Build history of the part. All positions in model axes, mm. A direction names the side the tool comes from. Give positions to 0.01 mm unless a question says otherwise; leave off trailing zeros. Write each loop counter-clockwise with the first axis right and the second up, starting at its lowest first coordinate (ties: lowest second). Pieces come first, ordered by that corner, then holes.
Autodesk Inventor part; units mm, degrees
ref_plane "YZ Plane" through (0, 0, 0) normal (1, 0, 0) x (0, 1, 0)
ref_plane "XZ Plane" through (0, 0, 0) normal (0, 1, 0) x (-1, 0, 0)
ref_plane "XY Plane" through (0, 0, 0) normal (0, 0, 1) x (1, 0, 0)
sketch "Sketch1" plane through (0, 0, 0) normal (0, 1, 0) x (-1, 0, 0)
  line L0 (-4, 0) -> (-157, 0)
  line L1 (-161, -4) -> (-161, -55)
  line L2 (-157, -59) -> (-4, -59)
  line L3 (0, -55) -> (0, -4)
  line L4 (-17, -3.5) -> (-62.5, -3.5)
  line L5 (-62.5, -3.5) -> (-62.5, -9.5)
  line L6 (-62.5, -9.5) -> (-17, -9.5)
  line L7 (-17, -9.5) -> (-17, -3.5)
  line L8 (-38, -15) -> (-64, -15)
  line L9 (-64, -15) -> (-64, -30)
  line L10 (-64, -30) -> (-38, -30)
  line L11 (-38, -30) -> (-38, -15)
  arc A0 (0, -4) -> (-4, 0) centre (-4, -4) ccw
  arc A1 (-157, 0) -> (-161, -4) centre (-157, -4) ccw
  arc A2 (-161, -55) -> (-157, -59) centre (-157, -55) ccw
  arc A3 (-4, -59) -> (0, -55) centre (-4, -55) ccw
  point P0 (0, 0)
  point P1 (-161, 0)
  point P2 (0, -59)
  dimension "d0" = 161
  dimension "d1" = 59
  dimension "d2" = 6
  dimension "d3" = 45.5
  dimension "d4" = 26
  dimension "d5" = 15
  dimension "d6" = 3.5
  dimension "d7" = 15
  dimension "d8" = 17
  dimension "d9" = 38
  dimension "d10" = 4
  dimension "d20" = 51
  dimension "d21" = 153
extrude "Extrusion1" add sketch "Sketch1" along normal blind 4.5
sketch "Sketch2" plane through (0, 4.5, 0) normal (0, 1, 0) x (1, 0, 0)
  line L0 (38, 15) -> (38, 30) construction
  line L1 (38, 30) -> (64, 30) construction
  line L2 (64, 30) -> (64, 15) construction
  line L3 (64, 15) -> (38, 15) construction
  line L4 (17, 3.5) -> (17, 9.5) construction
  line L5 (17, 9.5) -> (62.5, 9.5) construction
  line L6 (62.5, 9.5) -> (62.5, 3.5) construction
  line L7 (62.5, 3.5) -> (17, 3.5) construction
  line L8 (4, 0) -> (157, 0) construction
  arc A0 (157, 0) -> (161, 4) centre (157, 4) ccw construction
  line L9 (161, 4) -> (161, 55) construction
  arc A1 (161, 55) -> (157, 59) centre (157, 55) ccw construction
  line L10 (157, 59) -> (4, 59) construction
  arc A2 (4, 59) -> (0, 55) centre (4, 55) ccw construction
  line L11 (0, 55) -> (0, 4) construction
  arc A3 (0, 4) -> (4, 0) centre (4, 4) ccw construction
  point P0 (0, 0)
hole "Hole1" at (4, 4.5, -55) at (4, 4.5, -4) at (157, 4.5, -4) at (157, 4.5, -55) direction (0, -1, 0) diameter 3.5 end through all
properties part number "A8-0005"
(1) 3-axis set-ups, long thin cutter, end or side, ignore diameter. For faces 5 (the face through (82, 0, -29)), 6 (the face through (40, 2, -9.5)): which of +Z, -Z, +X, -X, +Y, -Y reach the whole face in a straight line?
(2) Saw through at C-C, the plane y = 1.2. List the corners of the cut face in (x, z), plus the area to 3 significant figures.
(3) Saw through at D-D, the plane x = 30.5. List the corners of the cut face in (y, z), plus the area to 4 significant figures.
(4) Mould opens along Z. For faces 1 (the face through (156.474, 2.218, -53.331)), 2 (the face through (39, 2, -3.5)), 3 (the face through (0, 2, -30)), 4 (the face through (159.797, 2.218, -57.859)) say: +Z half, -Z half, draft (parallel to the pull), parting line (faces both ways), or undercut.
(5) Probe line 1 (X direction, y = 2.6, z = -55); line 2 (Z direction, x = 4, y = 2.9); line 3 (X direction, y = 1.75, z = -4). List the from-to ranges inside material, lowest first.
(6) Saw through at B-B, the plane z = -24. List the corners of the cut face in (x, y), plus the area to 4 significant figures.
(7) Saw through at A-A, the plane x = 60. List the corners of the cut face in (y, z), plus the area to 3 significant figures.
(8) Drop a flat-ended pin along its axis: pin 1 (3 mm diameter, centred on x = 157, z = -55, fed in from -Y). Give the stop position or say it passes through.
Computed values:
1. face 5: +Z, -Z, +X, -X, -Y
1. face 6: +Y, -Y
2. outline: (0, -55) arc R4 ccw to (4, -59) - (157, -59) arc R4 ccw to (161, -55) - (161, -4) arc R4 ccw to (157, 0) - (4, 0) arc R4 ccw to (0, -4) - close; hole circle Ø3.5 at (4, -55); hole circle Ø3.5 at (4, -4); hole (17, -9.5) - (62.5, -9.5) - (62.5, -3.5) - (17, -3.5) - close; hole (38, -30) - (64, -30) - (64, -15) - (38, -15) - close; hole circle Ø3.5 at (157, -55); hole circle Ø3.5 at (157, -4)
2. area: 8,780 mm2
3. outline: (0, -59) - (4.5, -59) - (4.5, -9.5) - (0, -9.5) - close; (0, -3.5) - (4.5, -3.5) - (4.5, 0) - (0, 0) - close
3. area: 238.5 mm2
4. face 1: undercut
4. face 2: undercut
4. face 3: draft
4. face 4: -Z half
5. line 1: x = 0 to 2.25, 5.75 to 155.25, 158.75 to 161
5. line 2: z = -59 to -56.75, -53.25 to -5.75, -2.25 to 0
5. line 3: x = 0 to 2.25, 5.75 to 17, 62.5 to 155.25, 158.75 to 161
6. outline: (0, 0) - (38, 0) - (38, 4.5) - (0, 4.5) - close; (64, 0) - (161, 0) - (161, 4.5) - (64, 4.5) - close
6. area: 607.5 mm2
7. outline: (0, -59) - (4.5, -59) - (4.5, -30) - (0, -30) - close; (0, -15) - (4.5, -15) - (4.5, -9.5) - (0, -9.5) - close; (0, -3.5) - (4.5, -3.5) - (4.5, 0) - (0, 0) - close
7. area: 171 mm2
8. pin 1: passes through
